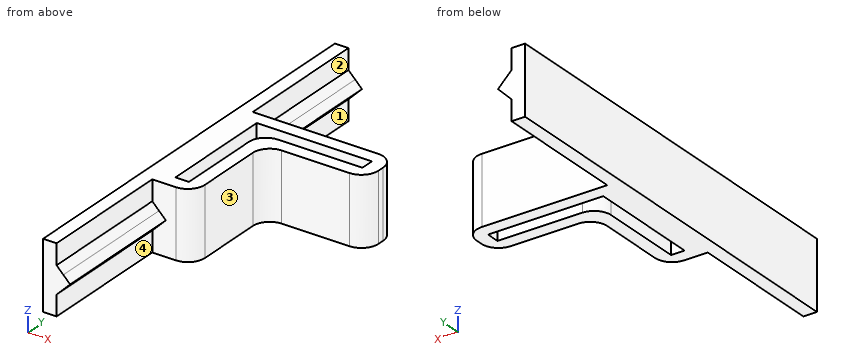
```python
from build123d import *

# Parameters (mm, degrees)
F1_DEPTH = 12.7
F2_R     = 3.175
F3_W     = 77.47
F3_H     = 12.7
F4_DEPTH = 2.54
F5_W     = 25.4
F5_H     = 2.54
F6_DEPTH = 2.54
F7_SIZE  = 1.26999


# Not quite as in the source:
# - a fillet or chamfer is up to 0.001 mm smaller than in the source, because OpenCascade refuses the exact size


with BuildPart() as f1:
    # F0 (on Top) → F1 (new body)
    with BuildSketch(Plane.XY):
        Polygon((0, 24.13), (0, -2.1948770154), (0, -2.54), (7.62, -2.54), (7.62, 16.51), (26.67, 16.51), (26.67, 24.13), align=None)
        Polygon((5.08, 0), (2.54, 0), (2.54, 21.59), (5.08, 21.59), (24.13, 21.59), (24.13, 19.05), (5.08, 19.05), align=None, mode=Mode.SUBTRACT)
    extrude(amount=F1_DEPTH)

    # F2
    f2_edges = [f1.edges().sort_by_distance(p)[0] for p in [
        (26.67, 24.13, 6.35),
        (26.67, 16.51, 6.35),
        (5.08, 19.05, 6.35),
        (7.62, -2.54, 6.35),
        (7.62, 16.51, 6.35),
    ]]
    fillet(f2_edges, radius=F2_R)

    # F3 (on face) → F4 (join)
    with BuildSketch(Plane(origin=(0, 0, 0), x_dir=(0, -1, 0), z_dir=(-1, 0, 0))):
        with Locations((-10.795, 6.35)):
            Rectangle(F3_W, F3_H)
    extrude(amount=F4_DEPTH)

    # F5 (on face) → F6 (join)
    with BuildSketch(Plane.YZ):
        with Locations((36.83, 6.35)):
            Rectangle(F5_W, F5_H)
        with Locations((-15.24, 6.35)):
            Rectangle(F5_W, F5_H)
    extrude(amount=F6_DEPTH)

    # F7 (size 1.27 in the source; OpenCascade refuses exactly that, so slightly less here)
    f7_edges = [f1.edges().sort_by_distance(p)[0] for p in [
        (2.54, -15.24, 5.08),
        (2.54, -15.24, 7.62),
        (2.54, 36.83, 7.62),
        (2.54, 36.83, 5.08),
        (0, -15.24, 5.08),
        (0, -15.24, 7.62),
        (0, 36.83, 7.62),
        (0, 36.83, 5.08),
    ]]
    chamfer(f7_edges, length=F7_SIZE)


solid = f1.part
```
Design review of the part built by this model. Coordinates are the model's own, in mm. Face numbers are marked on the shaded views. A direction names the side the tool comes from. Coordinates: 2 decimals unless noted, no trailing zeros. Order: outer loops, then holes, each group sorted by start corner. A loop starts at its lowest first (then second) coordinate and runs counter-clockwise, first axis right, second up.
1) Wall thickness on line 1 along Y through (x, z) = (15.75, 6); line 2 along X through (y, z) = (0.5, 12.25); line 3 along X through (y, z) = (14, 8.75): over which ranges is each line inside the solid? List them lowest first.
2) For the marked faces 1, 2, 3 and 4, list the 3-axis set-ups (+Z, -Z, +X, -X, +Y, -Y) from which the entire face can be reached by the end or side of a thin tool; tool diameter is ignored.
3) Clearance check with flat-ended pins moving along their axes: pin 1 (6 mm diameter, centred on x = 7, z = 11, fed in from -Y); pin 2 (4 mm diameter, centred on y = 39.5, z = 1.5, fed in from +X); pin 3 (4 mm diameter, centred on x = 8.5, z = 6, fed in from -Y). State where each tip first meets the part, or that it passes through.
4) Take a section at A-A, the plane x = 21.5. Give the boundary of the cut face in (y, z).
5) Take a section at B-B, the plane y = 5.5. Give the boundary of the cut face in (x, z), and give its area (3 significant figures).
Returned:
1. line 1: y = 16.51 to 19.05, 21.59 to 24.13
1. line 2: x = -2.54 to 2.54, 5.08 to 7.62
1. line 3: x = -2.54 to 2.54, 5.08 to 7.69
2. face 1: -Z, +X, +Y
2. face 2: +Z, +X, +Y
2. face 3: +Z, -Z, +X, -Y
2. face 4: -Z, +X, -Y
3. pin 1: stops at y = -2.54
3. pin 2: stops at x = 0
3. pin 3: stops at y = -1.79
4. outline: (16.51, 0) - (19.05, 0) - (19.05, 12.7) - (16.51, 12.7) - close; (21.59, 0) - (24.13, 0) - (24.13, 12.7) - (21.59, 12.7) - close
5. outline: (-2.54, 0) - (2.54, 0) - (2.54, 12.7) - (-2.54, 12.7) - close; (5.08, 0) - (7.62, 0) - (7.62, 12.7) - (5.08, 12.7) - close
5. area: 96.8 mm2
